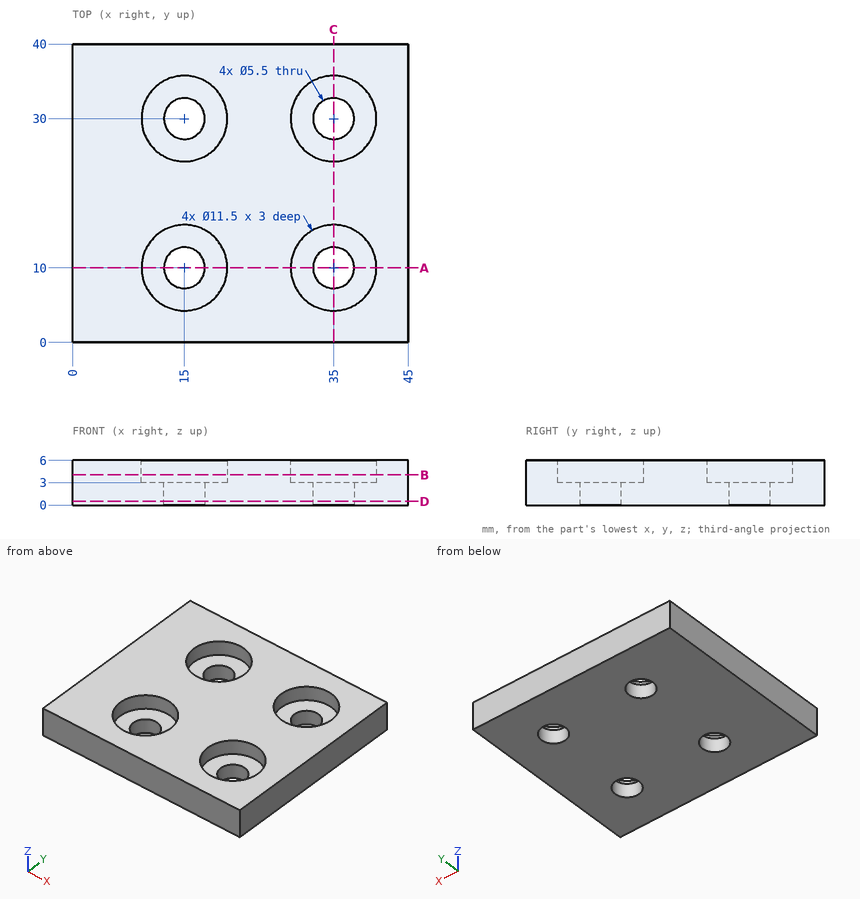
Could you check a few things on this drawing? It's one solid part, dimensions in mm from its lowest x, y, z. Coordinates: 2 decimals unless noted, no trailing zeros. Loops run counter-clockwise (first coordinate to the right, second up) from the corner with the lowest first, then second, coordinate; pieces in that order, holes last.
1. For P1, Ø7, axis at x = 35, y = 30, coming from the +Z side; P2, Ø9, axis at x = 15, y = 30, coming from the -Z side, each with a flat end and sliding along its axis, tell me the tip position at first contact or that it passes through.
2. Imagine slicing it at A-A (y = 10). Please give me the cut outline in (x, z).
3. Imagine slicing it at D-D (z = 0.5). Please give me the cut outline in (x, y), and give its area (3 significant figures).
4. I need wall thicknesses on L1, parallel to Y at x = 34.5, z = 4.65; L2, parallel to Y at x = 40, z = 3.9; L3, parallel to X at y = 13.5, z = 3.9. Which ranges of each line are inside material? Lowest first, please.
5. Imagine slicing it at B-B (z = 4.05). Please give me the cut outline in (x, y).
6. Imagine slicing it at C-C (x = 35). Please give me the cut outline in (y, z).
Computed values:
1. P1: stops at z = 3
1. P2: stops at z = 0
2. outline: (0, 0) - (12.25, 0) - (12.25, 3) - (9.25, 3) - (9.25, 6) - (0, 6) - close; (17.75, 0) - (32.25, 0) - (32.25, 3) - (29.25, 3) - (29.25, 6) - (20.75, 6) - (20.75, 3) - (17.75, 3) - close; (37.75, 0) - (45, 0) - (45, 6) - (40.75, 6) - (40.75, 3) - (37.75, 3) - close
3. outline: (0, 0) - (45, 0) - (45, 40) - (0, 40) - close; hole circle Ø5.5 at (15, 10); hole circle Ø5.5 at (15, 30); hole circle Ø5.5 at (35, 10); hole circle Ø5.5 at (35, 30)
3. area: 1,700 mm2
4. L1: y = 0 to 4.27, 15.73 to 24.27, 35.73 to 40
4. L2: y = 0 to 7.16, 12.84 to 27.16, 32.84 to 40
4. L3: x = 0 to 10.44, 19.56 to 30.44, 39.56 to 45
5. outline: (0, 0) - (45, 0) - (45, 40) - (0, 40) - close; hole circle Ø11.5 at (15, 10); hole circle Ø11.5 at (15, 30); hole circle Ø11.5 at (35, 10); hole circle Ø11.5 at (35, 30)
6. outline: (0, 0) - (7.25, 0) - (7.25, 3) - (4.25, 3) - (4.25, 6) - (0, 6) - close; (12.75, 0) - (27.25, 0) - (27.25, 3) - (24.25, 3) - (24.25, 6) - (15.75, 6) - (15.75, 3) - (12.75, 3) - close; (32.75, 0) - (40, 0) - (40, 6) - (35.75, 6) - (35.75, 3) - (32.75, 3) - close
